Geometry check sheet. Reference: the model listing, model coordinates, mm. A direction names the side the tool comes from. Round coordinates to 2 decimals unless told otherwise and drop trailing zeros. Write each loop counter-clockwise with the first axis right and the second up, starting at its lowest first coordinate (ties: lowest second). Pieces come first, ordered by that corner, then holes. Notation, with made-up numbers: (78, -7.75) - (130, -7.75) arc R27 cw to (130, 26.25) - close; hole circle Ø11 at (33.25, -29). An arc over 180 degrees is marked (long way). Return JSON: item names as keys, results as strings. Group by question number.
from build123d import *

# Parameters (mm, degrees)
SKETCH1_W           = 22
SKETCH1_H           = 12
BOSS_EXTRUDE1_DEPTH = 22.5
SKETCH2_W           = 12
SKETCH2_H           = 2
BOSS_EXTRUDE2_DEPTH = 5
CUT_EXTRUDE1_REACH  = 26.819
SKETCH4_R           = 6
BOSS_EXTRUDE3_DEPTH = 4
SKETCH5_R           = 2
BOSS_EXTRUDE4_DEPTH = 4
SKETCH6_R           = 2
BOSS_EXTRUDE5_DEPTH = 1.5
SKETCH7_R           = 3.5
BOSS_EXTRUDE6_DEPTH = 3.5
BOSS_EXTRUDE7_DEPTH = 1


with BuildPart() as part:
    # Sketch1 → Boss-Extrude1 (new body)
    with BuildSketch(Plane(origin=(0, 0, 0), x_dir=(1, 0, 0), z_dir=(0, 1, 0))):
        Rectangle(SKETCH1_W, SKETCH1_H)
    extrude(amount=BOSS_EXTRUDE1_DEPTH)

    # Sketch2 → Boss-Extrude2 (add)
    with BuildSketch(Plane.ZY.offset(11)):
        with Locations((0, 17)):
            Rectangle(SKETCH2_W, SKETCH2_H)
    boss_extrude2 = extrude(amount=BOSS_EXTRUDE2_DEPTH)

    # Sketch3 → Cut-Extrude1 (cut, up to next)
    with BuildSketch(Plane(origin=(0, 18, 0), x_dir=(1, 0, 0), z_dir=(0, 1, 0)), mode=Mode.PRIVATE) as cut_extrude1_sk1:
        with BuildLine():
            Line((-16, 0.5), (-16, -0.5))
            Line((-16, -0.5), (-15, -0.5))
            ThreePointArc((-15, -0.5), (-13, 0), (-15, 0.5))
            Line((-15, 0.5), (-16, 0.5))
        make_face()
    cut_extrude1_tool1 = extrude(cut_extrude1_sk1.sketch, amount=-CUT_EXTRUDE1_REACH, mode=Mode.PRIVATE) & part.part
    cut_extrude1 = cut_extrude1_tool1.solids().sort_by_distance((-14.365975, 18, 0))[0]
    add(cut_extrude1, mode=Mode.SUBTRACT)

    # Mirror1: Boss-Extrude2, Cut-Extrude1 across plane
    add(boss_extrude2.mirror(Plane(origin=(0, 0, 0), x_dir=(0, 0, 1), z_dir=(1, 0, 0))))
    add(cut_extrude1.mirror(Plane(origin=(0, 0, 0), x_dir=(0, 0, 1), z_dir=(1, 0, 0))), mode=Mode.SUBTRACT)

    # Sketch4 → Boss-Extrude3 (add)
    with BuildSketch(Plane(origin=(0, 22.5, 0), x_dir=(1, 0, 0), z_dir=(0, 1, 0))):
        with Locations(Location((-5, 0, 0), (0, 0, 270))):
            Circle(SKETCH4_R)
    extrude(amount=BOSS_EXTRUDE3_DEPTH)

    # Sketch5 → Boss-Extrude4 (add)
    with BuildSketch(Plane(origin=(0, 22.5, 0), x_dir=(1, 0, 0), z_dir=(0, 1, 0))):
        with Locations((2, 0)):
            Circle(SKETCH5_R)
    extrude(amount=BOSS_EXTRUDE4_DEPTH)

    # Sketch6 → Boss-Extrude5 (add)
    with BuildSketch(Plane(origin=(0, 26.5, 0), x_dir=(1, 0, 0), z_dir=(0, 1, 0))):
        with Locations(Location((-5, 0, 0), (0, 0, 270))):
            Circle(SKETCH6_R)
    extrude(amount=BOSS_EXTRUDE5_DEPTH)

    # Sketch7 → Boss-Extrude6 (add)
    with BuildSketch(Plane(origin=(0, 28, 0), x_dir=(1, 0, 0), z_dir=(0, 1, 0))):
        with Locations(Location((-5, 0, 0), (0, 0, 270))):
            Circle(SKETCH7_R)
    extrude(amount=BOSS_EXTRUDE6_DEPTH)

    # Sketch8 → Boss-Extrude7 (add)
    with BuildSketch(Plane(origin=(0, 31.5, 0), x_dir=(1, 0, 0), z_dir=(0, 1, 0))):
        with BuildLine():
            Line((-4.622076636, 3.479536453), (-4.622076636, -3.479536453))
            Line((-4.622076636, -3.479536453), (9, -2))
            ThreePointArc((9, -2), (11, 0), (9, 2))
            Line((9, 2), (-4.622076636, 3.479536453))
        make_face()
    extrude(amount=-BOSS_EXTRUDE7_DEPTH)


solid = part.part
1. Section check D-D (z = -4.75). Enter the section's corners in (x, y).
2. Section check A-A (x = 8.5). Enter the section's corners in (y, z), and give its area (3 significant figures).
3. Section check C-C (z = 2.5). Enter the section's corners in (x, y).
4. Depth check by flat-ended pin: pin 1 Ø2.5 at (x, z) = (-13, 3) entering from +Y; pin 2 Ø1.5 at (y, z) = (11, 0.5) entering from +X; pin 3 Ø2 at (y, z) = (24.5, 0.5) entering from +X. Enter the tip coordinate at first touch or a pass-through.
5. Mould release check, pull along Y, two halves, no side actions. Record for faces 1 (the face through (-12, 16, 0)), 2 (the face through (2.09, 31.01, 2.75)), 3 (the face through (-7, 27, 0)): pulls with the +Y half, pulls with the -Y half, needs draft (parallel to the pull), parting line crosses it, or undercut.
6. Tool access check on faces 4 (the face through (-11, 20, 0)), 5 (the face through (-11, 8, 0)), 6 (the face through (-7, 28, 2)). Record the directions out of +Z, -Z, +X, -X, +Y, -Y that give a thin tool (end or side, any length) a straight path to the whole face; none if there is none.
7. Section check B-B (y = 16.5). Enter the section's corners in (x, z) (1 decimal), and give its area (3 significant figures).
8. Material ranges on line 1 along Y through (x, z) = (3.5, 0.5); line 2 along Y through (x, z) = (8.5, 0); line 3 along X through (y, z) = (10.5, -3.25), recorded low to high.
Result sheet:
{
 "1": {"outline": "(-16, 16) - (-11, 16) - (-11, 0) - (11, 0) - (11, 16) - (16, 16) - (16, 18) - (11, 18) - (11, 22.5) - (-1.33, 22.5) - (-1.33, 26.5) - (-8.67, 26.5) - (-8.67, 22.5) - (-11, 22.5) - (-11, 18) - (-16, 18) - close"},
 "2": {"outline": "(0, -6) - (22.5, -6) - (22.5, 6) - (0, 6) - close; (30.5, -2.05) - (31.5, -2.05) - (31.5, 2.05) - (30.5, 2.05) - close", "area": "274 mm²"},
 "3": {"outline": "(-16, 16) - (-11, 16) - (-11, 0) - (11, 0) - (11, 16) - (16, 16) - (16, 18) - (11, 18) - (11, 22.5) - (0.45, 22.5) - (0.45, 26.5) - (-10.45, 26.5) - (-10.45, 22.5) - (-11, 22.5) - (-11, 18) - (-16, 18) - close; (-7.45, 28) - (-2.55, 28) - (-2.55, 30.5) - (4.4, 30.5) - (4.4, 31.5) - (-7.45, 31.5) - close"},
 "4": {"pin 1": "stops at y = 18", "pin 2": "stops at x = 11", "pin 3": "stops at x = 4"},
 "5": {"face 1": "pulls with the -Y half", "face 2": "needs draft", "face 3": "undercut"},
 "6": {"face 4": "+Z, -Z, -X, +Y", "face 5": "+Z, -Z, -X, -Y", "face 6": "none"},
 "7": {"outline": "(-16, -6) - (16, -6) - (16, -0.5) - (15, -0.5) arc R1.1 cw (long way) to (15, 0.5) - (16, 0.5) - (16, 6) - (-16, 6) - (-16, 0.5) - (-15, 0.5) arc R1.1 cw (long way) to (-15, -0.5) - (-16, -0.5) - close", "area": "375 mm²"},
 "8": {"line 1": "y = 0 to 26.5, 30.5 to 31.5", "line 2": "y = 0 to 22.5, 30.5 to 31.5", "line 3": "x = -11 to 11"}
}
